Autodesk Inventor part; units mm, degrees
ref_plane "HUELSE3_1_XY" through (11, 1.4, -14) normal (1, 0, 0) x (0, 0, -1)
ref_plane "HUELSE3_1_YZ" through (11, 1.4, -14) normal (0, 0, -1) x (0, 1, 0)
ref_plane "HUELSE3_1_ZX" through (11, 1.4, -14) normal (0, 1, 0) x (1, 0, 0)
sketch "Skizze_1" plane through (12, 0, 0) normal (1, 0, 0) x (0, 0, -1)
  line L0 (-32.5, -14) -> (-31.5, -15)
  line L1 (-31.5, -15) -> (31.5, -15)
  line L2 (31.5, -15) -> (32.5, -14)
  line L3 (32.5, -14) -> (32.5, 14)
  line L4 (32.5, 14) -> (31.5, 15)
  line L5 (31.5, 15) -> (-31.5, 15)
  line L6 (-31.5, 15) -> (-32.5, 14)
  line L7 (-32.5, 14) -> (-32.5, -14)
extrude "Extrusion1" add sketch "Skizze_1" against normal blind 10
sketch "Skizze_2" plane through (0, 0, 0) normal (0, 1, 0) x (1, 0, 0)
  line L0 (-252, -23) -> (2, -23)
  line L1 (2, -23) -> (2, -28)
  line L2 (2, -28) -> (-251, -28)
  line L3 (-251, -28) -> (-252, -27.4226)
  line L4 (-252, -27.4226) -> (-252, -23)
  line L5 (-252, -23) -> (2, -23)
sketch "Skizze_3" plane through (0, 0, 0) normal (0, 1, 0) x (1, 0, 0)
  line L0 (-252, 23) -> (2, 23)
  line L1 (2, 23) -> (2, 18)
  line L2 (2, 18) -> (-251, 18)
  line L3 (-251, 18) -> (-252, 18.5774)
  line L4 (-252, 18.5774) -> (-252, 23)
  line L5 (-252, 23) -> (2, 23)
sketch "Skizze_4" plane through (0, -8.6, 0) normal (0, 1, 0) x (1, 0, 0)
  line L0 (12, -10) -> (2, -10)
  line L1 (2, -10) -> (2, -7.5)
  line L2 (2, -7.5) -> (2.433, -7.933)
  line L3 (2.433, -7.933) -> (11.567, -7.933)
  line L4 (11.567, -7.933) -> (12, -7.5)
  line L5 (12, -7.5) -> (12, -10)
  line L6 (12, -10) -> (2, -10)
revolve "Revolution1" cut sketch "Skizze_4" angle 360 about axis through (12, -8.6, 10) along (1, 0, 0)
thread "Thread1"
sketch "Skizze_5" plane through (0, -8.6, 0) normal (0, 1, 0) x (1, 0, 0)
  line L0 (12, 10) -> (2, 10)
  line L1 (2, 10) -> (2, 12.5)
  line L2 (2, 12.5) -> (2.433, 12.067)
  line L3 (2.433, 12.067) -> (11.567, 12.067)
  line L4 (11.567, 12.067) -> (12, 12.5)
  line L5 (12, 12.5) -> (12, 10)
  line L6 (12, 10) -> (2, 10)
revolve "Revolution2" cut sketch "Skizze_5" angle 360 about axis through (12, -8.6, -10) along (1, 0, 0)
thread "Thread2"
sketch "Skizze_6" plane through (0, 11.4, 0) normal (0, 1, 0) x (1, 0, 0)
  line L0 (12, -10) -> (2, -10)
  line L1 (2, -10) -> (2, -7.5)
  line L2 (2, -7.5) -> (2.433, -7.933)
  line L3 (2.433, -7.933) -> (11.567, -7.933)
  line L4 (11.567, -7.933) -> (12, -7.5)
  line L5 (12, -7.5) -> (12, -10)
  line L6 (12, -10) -> (2, -10)
revolve "Revolution3" cut sketch "Skizze_6" angle 360 about axis through (12, 11.4, 10) along (1, 0, 0)
thread "Thread3"
sketch "Skizze_7" plane through (0, 11.4, 0) normal (0, 1, 0) x (1, 0, 0)
  line L0 (12, 10) -> (2, 10)
  line L1 (2, 10) -> (2, 12.5)
  line L2 (2, 12.5) -> (2.433, 12.067)
  line L3 (2.433, 12.067) -> (11.567, 12.067)
  line L4 (11.567, 12.067) -> (12, 12.5)
  line L5 (12, 12.5) -> (12, 10)
  line L6 (12, 10) -> (2, 10)
revolve "Revolution4" cut sketch "Skizze_7" angle 360 about axis through (12, 11.4, -10) along (1, 0, 0)
thread "Thread4"
sketch "Skizze_8" plane through (0, 0, 0) normal (0, 0, 1) x (1, 0, 0)
  line L0 (2, 0) -> (-181.95, 0)
  line L1 (-181.95, 0) -> (-181.95, 8)
  line L2 (-181.95, 8) -> (-173.95, 8)
  line L3 (-173.95, 8) -> (-173.95, 3)
  line L4 (-173.95, 3) -> (2, 3)
  line L5 (2, 3) -> (2, 0)
  line L6 (2, 0) -> (-181.95, 0)
revolve "Revolution5" add sketch "Skizze_8" angle 360 about axis through (2, 0, 0) along (1, 0, 0)
sketch "Sketch9" plane through (12, 15, 31.5) normal (0, 1, 0) x (1, 0, 0)
  point P0 (-5, 8.5)
hole "Hole1" at (7, 15, 23) direction (0, -1, 0) diameter 3.242 depth 15 countersink diameter 4 countersink angle 90
sketch "Sketch10" plane through (12, 15, 31.5) normal (0, 1, 0) x (1, 0, 0)
  point P0 (-5, 54.5)
hole "Hole2" at (7, 15, -23) direction (0, -1, 0) diameter 3.242 depth 15 countersink diameter 4 countersink angle 90
revolve "Revolution6" add sketch "Skizze_2" angle 360 about axis through (-252, 0, 23) along (-1, 0, 0)
revolve "Revolution7" add sketch "Skizze_3" angle 360 about axis through (-252, 0, -23) along (-1, 0, 0)
sketch "Sketch11" plane through (12, 0, 0) normal (1, 0, 0) x (0, 0, -1)
  point P0 (14, 1.4)
hole "Hole3" at (12, 1.4, -14) direction (-1, 0, 0) diameter 5 depth 1 tip angle 120
sketch "Sketch12" plane through (12, 0, 0) normal (1, 0, 0) x (0, 0, -1)
  point P0 (-14, 1.4)
hole "Hole4" at (12, 1.4, 14) direction (-1, 0, 0) diameter 5 depth 1 tip angle 120
sketch "Sketch_4" plane through (0, 0, 0) normal (0, 1, 0) x (1, 0, 0)
  line L0 (12, 23) -> (11.65, 23)
  line L1 (11.65, 23) -> (11.65, 26.4725)
  arc A0 (11.65, 26.4725) -> (11.1936, 26.9706) centre (11.15, 26.4725) ccw
  line L2 (11.1936, 26.9706) -> (8, 27.25)
  line L3 (8, 27.25) -> (8, 28)
  line L4 (8, 28) -> (12, 28)
  line L5 (12, 28) -> (12, 23)
  line L6 (12, 23) -> (11.65, 23)
revolve "Revolution8" cut sketch "Sketch_4" angle 360 about axis through (12, 0, -23) along (1, 0, 0)
sketch "Sketch_6" plane through (0, 0, 0) normal (0, 1, 0) x (1, 0, 0)
  line L0 (12, -23) -> (11.65, -23)
  line L1 (11.65, -23) -> (11.65, -19.5275)
  arc A0 (11.65, -19.5275) -> (11.1936, -19.0294) centre (11.15, -19.5275) ccw
  line L2 (11.1936, -19.0294) -> (8, -18.75)
  line L3 (8, -18.75) -> (8, -18)
  line L4 (8, -18) -> (12, -18)
  line L5 (12, -18) -> (12, -23)
  line L6 (12, -23) -> (11.65, -23)
revolve "Revolution9" cut sketch "Sketch_6" angle 360 about axis through (12, 0, 23) along (1, 0, 0)
sketch "Sketch_7" plane through (11.65, 0, 23) normal (1, 0, 0) x (0, 0, -1)
  arc A0 (-1.8677, -0.5727) -> (-1.4298, -1.3311) centre (-1.5588, -0.9) ccw
  arc A1 (-0.4379, -1.9038) -> (-1.4298, -1.3311) centre (-1.2041, -2.0855) ccw
  arc A2 (-0.4379, -1.9038) -> (0.4379, -1.9038) centre (0, -1.8) ccw
  arc A3 (1.4298, -1.3311) -> (0.4379, -1.9038) centre (1.2041, -2.0855) ccw
  arc A4 (1.4298, -1.3311) -> (1.8677, -0.5727) centre (1.5588, -0.9) ccw
  arc A5 (1.8677, 0.5727) -> (1.8677, -0.5727) centre (2.4082, 0) ccw
  arc A6 (1.8677, 0.5727) -> (1.4298, 1.3311) centre (1.5588, 0.9) ccw
  arc A7 (0.4379, 1.9038) -> (1.4298, 1.3311) centre (1.2041, 2.0855) ccw
  arc A8 (0.4379, 1.9038) -> (-0.4379, 1.9038) centre (0, 1.8) ccw
  arc A9 (-1.4298, 1.3311) -> (-0.4379, 1.9038) centre (-1.2041, 2.0855) ccw
  arc A10 (-1.4298, 1.3311) -> (-1.8677, 0.5727) centre (-1.5588, 0.9) ccw
  arc A11 (-1.8677, -0.5727) -> (-1.8677, 0.5727) centre (-2.4082, 0) ccw
extrude "Extrusion2" cut sketch "Sketch_7" against normal blind 2.48
sketch "Sketch_8" plane through (11.65, 0, -23) normal (1, 0, 0) x (0, 0, -1)
  arc A0 (-1.8677, -0.5727) -> (-1.4298, -1.3311) centre (-1.5588, -0.9) ccw
  arc A1 (-0.4379, -1.9038) -> (-1.4298, -1.3311) centre (-1.2041, -2.0855) ccw
  arc A2 (-0.4379, -1.9038) -> (0.4379, -1.9038) centre (0, -1.8) ccw
  arc A3 (1.4298, -1.3311) -> (0.4379, -1.9038) centre (1.2041, -2.0855) ccw
  arc A4 (1.4298, -1.3311) -> (1.8677, -0.5727) centre (1.5588, -0.9) ccw
  arc A5 (1.8677, 0.5727) -> (1.8677, -0.5727) centre (2.4082, 0) ccw
  arc A6 (1.8677, 0.5727) -> (1.4298, 1.3311) centre (1.5588, 0.9) ccw
  arc A7 (0.4379, 1.9038) -> (1.4298, 1.3311) centre (1.2041, 2.0855) ccw
  arc A8 (0.4379, 1.9038) -> (-0.4379, 1.9038) centre (0, 1.8) ccw
  arc A9 (-1.4298, 1.3311) -> (-0.4379, 1.9038) centre (-1.2041, 2.0855) ccw
  arc A10 (-1.4298, 1.3311) -> (-1.8677, 0.5727) centre (-1.5588, 0.9) ccw
  arc A11 (-1.8677, -0.5727) -> (-1.8677, 0.5727) centre (-2.4082, 0) ccw
extrude "Extrusion3" cut sketch "Sketch_8" against normal blind 2.48
sketch "Sketch_9" plane through (0, 0, 0) normal (0, 0, 1) x (1, 0, 0)
  line L0 (12, 0) -> (9.868, 0)
  line L1 (9.868, 0) -> (11.6, 1.732)
  line L2 (11.6, 1.732) -> (11.6, 3.1)
  arc A0 (11.6, 3.1) -> (11.2, 3.5) centre (11.2, 3.1) ccw
  line L3 (11.2, 3.5) -> (7.6, 3.5)
  line L4 (7.6, 3.5) -> (7.6, 4)
  line L5 (7.6, 4) -> (12, 4)
  line L6 (12, 4) -> (12, 0)
  line L7 (12, 0) -> (9.868, 0)
revolve "Revolution10" cut sketch "Sketch_9" angle 360 about axis through (12, 0, 0) along (1, 0, 0)
sketch "Sketch_10" plane through (11.6, 0, 0) normal (1, 0, 0) x (0, 1, 0)
  line L0 (-1.5, -0.866) -> (0, -1.7321)
  line L1 (0, -1.7321) -> (1.5, -0.866)
  line L2 (1.5, -0.866) -> (1.5, 0.866)
  line L3 (1.5, 0.866) -> (0, 1.7321)
  line L4 (0, 1.7321) -> (-1.5, 0.866)
  line L5 (-1.5, 0.866) -> (-1.5, -0.866)
extrude "Extrusion4" cut sketch "Sketch_10" against normal blind 2
ref_plane "HUELSE3_1_XY" through (11, 1.4, -14) normal (1, 0, 0) x (0, 0, -1)
ref_plane "HUELSE3_1_YZ" through (11, 1.4, -14) normal (0, 0, -1) x (0, 1, 0)
ref_plane "HUELSE3_1_ZX" through (11, 1.4, -14) normal (0, 1, 0) x (1, 0, 0)
ref_plane "HUELSE3_2_XY" through (11, 1.4, 14) normal (1, 0, 0) x (0, 0, -1)
ref_plane "HUELSE3_2_YZ" through (11, 1.4, 14) normal (0, 0, -1) x (0, 1, 0)
ref_plane "HUELSE3_2_ZX" through (11, 1.4, 14) normal (0, 1, 0) x (1, 0, 0)
ref_plane "kolben_dfm_XY" through (0, 0, 0) normal (-1, 0, 0) x (0, 0, -1)
ref_plane "kolben_dfm_YZ" through (0, 0, 0) normal (0, 0, -1) x (0, -1, 0)
ref_plane "kolben_dfm_ZX" through (0, 0, 0) normal (0, -1, 0) x (-1, 0, 0)
properties part number "529120 DFM-16-160-B-P-A-KF---(K)"
Check sheet for the modelled part. Datum: model origin and axes. Units: mm. A direction names the side the tool comes from. Coordinates: 2 decimals unless noted, no trailing zeros. Loops run counter-clockwise (first coordinate to the right, second up) from the corner with the lowest first, then second, coordinate; pieces in that order, holes last.
1) Release check for a two-part mould opening along X. For faces 4 (the face through (-85, -3, 0)), 5 (the face through (7, -15, 0)), 6 (the face through (9.929, -3.441, -25.194)) record: released by +X, released by -X, zero draft, split by the parting line, or undercut.
2) Sectioned sample at A-A (x = -187). Record the boundary of the cut face in (y, z).
3) Access from +Z, -Z, +X, -X, +Y, -Y to the whole of each face (thin tool, end or side, straight path). Record for faces 1 (the face through (9.375, 3.233, 1.341)), 2 (the face through (7.06, -9.86, -8.36)), 3 (the face through (-126, 0, 18)).
4) Gauge pin test, flat ends, axial feed: pin 1 (3 mm diameter, centred on y = -0.5, z = 21.5, fed in from +X); pin 2 (1.5 mm diameter, centred on x = -138.5, z = 21, fed in from +Y); pin 3 (8 mm diameter, centred on x = -104, z = -21, fed in from +Y); pin 4 (8 mm diameter, centred on x = -99, z = -9, fed in from +Y). Record the tip position at first contact, or that the pin passes through.
5) Material ranges on probe 1 along Y at (x, z) = (5.25, 10); probe 2 along Z at (x, y) = (7, 9); probe 3 along Y at (x, z) = (11, -14), recorded low to high.
Check sheet entries:
1. face 4: undercut
1. face 5: zero draft
1. face 6: released by +X
2. outline: circle Ø10 at (0, -23); circle Ø10 at (0, 23)
3. face 1: +X
3. face 2: +X, -X
3. face 3: -X
4. pin 1: stops at x = 11.65
4. pin 2: stops at y = 4.84
4. pin 3: stops at y = 5
4. pin 4: passes through
5. probe 1: y = -15 to -10.67, -6.53 to 9.33, 13.47 to 15
5. probe 2: z = -32.5 to -24.62, -21.38 to 21.38, 24.62 to 32.5
5. probe 3: y = -15 to -1.1, 3.9 to 15
